Part print with two shaded views. Sizes in mm from the minimum x, y, z corner. Round coordinates to 2 decimals unless told otherwise and drop trailing zeros. Order: outer loops, then holes, each group sorted by start corner. A loop starts at its lowest first (then second) coordinate and runs counter-clockwise, first axis right, second up. Notation, with made-up numbers: (75, 84) - (89, 84) arc R27 ccw to (89, 119) - close; hole circle Ø6 at (83.5, 4). An arc over 180 degrees is marked (long way). Use one line per item in the form item = value.
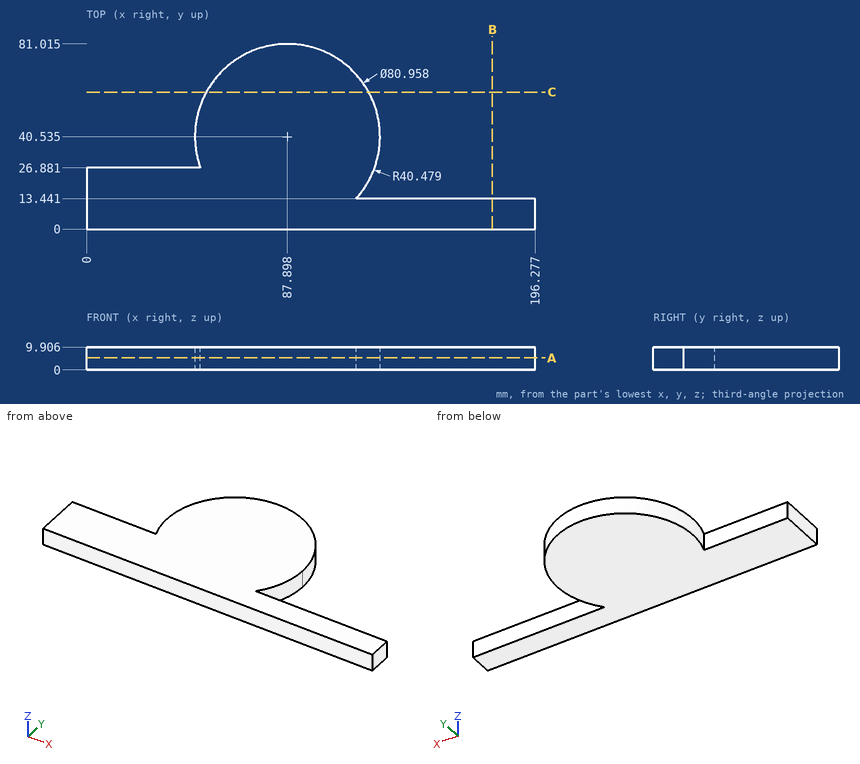
(1) Probe probe 1 along Y at (x, z) = (149, 8.25); probe 2 along Y at (x, z) = (21, 8.75); probe 3 along X at (y, z) = (41.5, 2.25) (1 decimal). List the from-to ranges inside material, lowest first. Write a range as [from, to].
Report:
probe_1 = [0, 13.44]
probe_2 = [0, 26.88]
probe_3 = [47.4, 128.4]
(2) Slice it at B-B on x = 177.5. Give the cut face in (y, z).
Report:
outline = (0, 0) - (13.44, 0) - (13.44, 9.91) - (0, 9.91) - close
(3) Slice it at C-C on y = 60. Give the cut face in (x, z) (1 decimal), then the cut area to 3 significant figures.
Report:
outline = (52.4, 0) - (123.4, 0) - (123.4, 9.9) - (52.4, 9.9) - close
area = 703 mm2
(4) Pin check, flat tips, straight feed: pin 1 (1 mm diameter, centred on y = 47, z = 3.5, fed in from -X); pin 2 (3 mm diameter, centred on x = 170, z = 6, fed in from +Y); pin 3 (3 mm diameter, centred on x = 24.5, z = 6, fed in from +Y). Stop position of each tip, or through.
Report:
pin_1 = 47.86
pin_2 = 13.44
pin_3 = 26.88
(5) Slice it at A-A on z = 5.25. Give the cut face in (x, y) (1 decimal).
Report:
outline = (0, 0) - (196.3, 0) - (196.3, 13.4) - (118, 13.4) arc R40.5 ccw (long way) to (49.8, 26.9) - (0, 26.9) - close
